Could you check a few things on this model? Use its own coordinates, in mm. A direction names the side the tool comes from. Coordinates: 2 decimals unless noted, no trailing zeros. Write each loop counter-clockwise with the first axis right and the second up, starting at its lowest first coordinate (ties: lowest second). Pieces come first, ordered by that corner, then holes. Notation, with made-up numbers: (-38.5, -17) - (18.5, -17) arc R12 ccw to (18.5, -1) - close; hole circle Ø8 at (49.25, 38). An arc over 180 degrees is marked (long way). Write item = value, one per line. Start each with the question number.
```python
from build123d import *

# Parameters (mm, degrees)
SKETCH_1_R      = 2.25
SKETCH_1_R_2    = 9.5
SKETCH_1_R_3    = 2
EXTRUDE_1_DEPTH = 4


with BuildPart() as part:
    # 草图1 → 凸台-拉伸1 (new body)
    with BuildSketch(Plane.XY):
        Polygon((0, 4.863043478), (-4, 4.863043478), (-4, 12.863043478), (0, 12.863043478), (0, 22.363043478), (4, 22.363043478), (4, 21.013043478), (6.6, 21.013043478), (6.6, 22.363043478), (8.6, 22.363043478), (8.6, 25.363043478), (6.6, 25.363043478), (6.6, 26.713043478), (4, 26.713043478), (4, 25.363043478), (0, 25.363043478), (0, 31.363043478), (70, 31.363043478), (70, 25.363043478), (66, 25.363043478), (66, 26.713043478), (63.4, 26.713043478), (63.4, 25.363043478), (61.4, 25.363043478), (61.4, 22.363043478), (63.4, 22.363043478), (63.4, 21.013043478), (66, 21.013043478), (66, 22.363043478), (70, 22.363043478), (70, 12.863043478), (74, 12.863043478), (74, 4.863043478), (70, 4.863043478), (70, -4.636956522), (66, -4.636956522), (66, -3.286956522), (63.4, -3.286956522), (63.4, -4.636956522), (61.4, -4.636956522), (61.4, -7.636956522), (63.4, -7.636956522), (63.4, -8.986956522), (66, -8.986956522), (66, -7.636956522), (70, -7.636956522), (70, -17.136956522), (74, -17.136956522), (74, -25.136956522), (70, -25.136956522), (70, -77.136956522), (74, -77.136956522), (74, -85.136956522), (70, -85.136956522), (70, -94.636956522), (66, -94.636956522), (66, -93.286956522), (63.4, -93.286956522), (63.4, -94.636956522), (61.4, -94.636956522), (61.4, -97.636956522), (63.4, -97.636956522), (63.4, -98.986956522), (66, -98.986956522), (66, -97.636956522), (70, -97.636956522), (70, -117.636956522), (0, -117.636956522), (0, -97.636956522), (4, -97.636956522), (4, -98.986956522), (6.6, -98.986956522), (6.6, -97.636956522), (8.6, -97.636956522), (8.6, -94.636956522), (6.6, -94.636956522), (6.6, -93.286956522), (4, -93.286956522), (4, -94.636956522), (0, -94.636956522), (0, -85.136956522), (-4, -85.136956522), (-4, -77.136956522), (0, -77.136956522), (0, -25.136956522), (-4, -25.136956522), (-4, -17.136956522), (0, -17.136956522), (0, -7.636956522), (4, -7.636956522), (4, -8.986956522), (6.6, -8.986956522), (6.6, -7.636956522), (8.6, -7.636956522), (8.6, -4.636956522), (6.6, -4.636956522), (6.6, -3.286956522), (4, -3.286956522), (4, -4.636956522), (0, -4.636956522), align=None)
        with Locations((35, 8.863043478)):
            Circle(SKETCH_1_R, mode=Mode.SUBTRACT)
        with Locations((35, -51.136956522)):
            Circle(SKETCH_1_R_2, mode=Mode.SUBTRACT)
        with Locations((55, -51.136956522)):
            Circle(SKETCH_1_R_3, mode=Mode.SUBTRACT)
        with Locations(Location((15, -51.136956522, 0), (0, 0, 180))):
            Circle(SKETCH_1_R_3, mode=Mode.SUBTRACT)
        with Locations((55, -91.136956522)):
            Circle(SKETCH_1_R_3, mode=Mode.SUBTRACT)
        with Locations(Location((15, -91.136956522, 0), (0, 0, 180))):
            Circle(SKETCH_1_R_3, mode=Mode.SUBTRACT)
    extrude(amount=EXTRUDE_1_DEPTH)


solid = part.part
```
1) Thinking about a two-plate mould opening in Y: for faces 5 (the flat face through (70, -12, 2)), 6 (the flat face through (-2, 12.863, 2)), 7 (the flat face through (-4, 9, 2)), which applies, +Y half, -Y half, draft (parallel to the pull), parting line (faces both ways), or undercut?
2) Suppose I cut it at D-D on y = -108. Please give me the cut outline in (x, z), plus the area to 3 significant figures.
3) Which directions (+Z, -Z, +X, -X, +Y, -Y) give clear straight access to the entire face, cutting with the end or side of a thin tool? Please do faces 1 (the flat face through (0, -108, 2)), 2 (the flat face through (2, 22.363, 2)), 3 (the flat face through (68, -94.637, 2)), 4 (the flat face through (72, -85.137, 2)).
4) If I drill on probe 1 along Y at (x, z) = (3, 3.1); probe 2 along Y at (x, z) = (15, 0.9); probe 3 along X at (y, z) = (-91, 3.7), over which ranges is the centre line in solid material (lowest first)? Write a range as [from, to].
5) Suppose I cut it at B-B on x = 35. Please give me the cut outline in (y, z).
6) For P1, Ø2, axis at y = 1.5, z = 1.5, coming from the -X side; P2, Ø3, axis at x = 15, y = -51.14, coming from the +Z side, each with a flat end and sliding along its axis, tell me the tip position at first contact or that it passes through.
7) Suppose I cut it at C-C on z = 1.75. State how many separate pieces and enclosed holes the cut face has, plus the area to 3 significant figures.
8) Suppose I cut it at A-A on x = 55. Please give me the cut outline in (y, z).
Reply:
q1.face_5 = undercut
q1.face_6 = +Y half
q1.face_7 = draft
q2.outline = (0, 0) - (70, 0) - (70, 4) - (0, 4) - close
q2.area = 280 mm^2
q3.face_1 = +Z, -Z, -X, -Y
q3.face_2 = +Z, -Z, -X
q3.face_3 = +Z, -Z, +X
q3.face_4 = +Z, -Z, +X, -Y
q4.probe_1 = [-117.64, -97.64], [-94.64, -7.64], [-4.64, 22.36], [25.36, 31.36]
q4.probe_2 = [-117.64, -93.14], [-89.14, -53.14], [-49.14, 31.36]
q4.probe_3 = [0, 13], [17, 53], [57, 70]
q5.outline = (-117.64, 0) - (-60.64, 0) - (-60.64, 4) - (-117.64, 4) - close; (-41.64, 0) - (6.61, 0) - (6.61, 4) - (-41.64, 4) - close; (11.11, 0) - (31.36, 0) - (31.36, 4) - (11.11, 4) - close
q6.P1 = 0
q6.P2 = through
q7.separate_pieces = 1
q7.enclosed_holes = 6
q7.area = 10,100 mm^2
q8.outline = (-117.64, 0) - (-93.14, 0) - (-93.14, 4) - (-117.64, 4) - close; (-89.14, 0) - (-53.14, 0) - (-53.14, 4) - (-89.14, 4) - close; (-49.14, 0) - (31.36, 0) - (31.36, 4) - (-49.14, 4) - close
